Geometry check sheet. Reference: the model listing, model coordinates, mm. Face numbers are marked on the shaded views. A direction names the side the tool comes from. Give positions to 0.01 mm unless a question says otherwise; leave off trailing zeros. Loops run counter-clockwise (first coordinate to the right, second up) from the corner with the lowest first, then second, coordinate; pieces in that order, holes last.
1. Cross-section at D-D, the plane z = 1.25. Record the cut outline in (x, y).
2. Tool access check on the marked faces 1, 2 and 3. Record the directions out of +Z, -Z, +X, -X, +Y, -Y that give a thin tool (end or side, any length) a straight path to the whole face; none if there is none.
3. Cross-section at B-B, the plane y = 20. Record the cut outline in (x, z) (3 decimals).
4. Material ranges on L1, parallel to X at y = 10, z = 9 (3 decimals); L2, parallel to X at y = 14, z = 4; L3, parallel to X at y = 3.75, z = 9.5, recorded low to high.
5. Release check for a two-part mould opening along Z. For the marked faces 4, 5 and 6 record: +Z half, -Z half, draft (parallel to the pull), parting line (faces both ways), or undercut.
6. Cross-section at C-C, the plane x = 48.5. Record the cut outline in (y, z) (3 decimals), plus the area to 3 significant figures.
7. Cross-section at A-A, the plane z = 9. State how many separate pieces and enclosed holes the cut face has, plus the area to 3 significant figures.
from build123d import *

# Parameters (mm, degrees)
SKETCH1_W           = 75
SKETCH1_H           = 18
BOSS_EXTRUDE1_DEPTH = 24
SKETCH2_W           = 36
SKETCH2_H           = 18
CUT_EXTRUDE1_DEPTH  = 20
CUT_EXTRUDE2_REACH  = 81.681
SKETCH3_R           = 2.075
CUT_EXTRUDE4_REACH  = 82.777
SKETCH4_R           = 3.075
CUT_EXTRUDE5_DEPTH  = 5


with BuildPart() as part:
    # Sketch1 → Boss-Extrude1 (new body)
    with BuildSketch(Plane(origin=(0, 0, 0), x_dir=(1, 0, 0), z_dir=(0, 1, 0))):
        with Locations((37.5, -9)):
            Rectangle(SKETCH1_W, SKETCH1_H)
    extrude(amount=BOSS_EXTRUDE1_DEPTH)

    # Sketch2 → Cut-Extrude1 (cut)
    with BuildSketch(Plane(origin=(0, 24, 0), x_dir=(1, 0, 0), z_dir=(0, 1, 0))):
        with Locations((37.5, -9)):
            Rectangle(SKETCH2_W, SKETCH2_H)
    extrude(amount=-CUT_EXTRUDE1_DEPTH, mode=Mode.SUBTRACT)

    # Sketch3 → Cut-Extrude2 (cut, up to next)
    with BuildSketch(Plane(origin=(0, 4, 0), x_dir=(1, 0, 0), z_dir=(0, 1, 0)), mode=Mode.PRIVATE) as cut_extrude2_sk1:
        with Locations(Location((26.5, -9, 0), (0, 0, 270))):
            Circle(SKETCH3_R)
    cut_extrude2_tool1 = extrude(cut_extrude2_sk1.sketch, amount=-CUT_EXTRUDE2_REACH, mode=Mode.PRIVATE) & part.part
    # Sketch3 → Cut-Extrude2 (cut, up to next)
    with BuildSketch(Plane(origin=(0, 4, 0), x_dir=(1, 0, 0), z_dir=(0, 1, 0)), mode=Mode.PRIVATE) as cut_extrude2_sk2:
        with Locations(Location((48.5, -9, 0), (0, 0, 270))):
            Circle(SKETCH3_R)
    cut_extrude2_tool2 = extrude(cut_extrude2_sk2.sketch, amount=-CUT_EXTRUDE2_REACH, mode=Mode.PRIVATE) & part.part
    add(cut_extrude2_tool1.solids().sort_by_distance((26.5, 4, 9))[0], mode=Mode.SUBTRACT)
    add(cut_extrude2_tool2.solids().sort_by_distance((48.5, 4, 9))[0], mode=Mode.SUBTRACT)

    # Sketch4 → Cut-Extrude4 (cut, up to next)
    with BuildSketch(Plane(origin=(0, 24, 0), x_dir=(1, 0, 0), z_dir=(0, 1, 0)), mode=Mode.PRIVATE) as cut_extrude4_sk1:
        with Locations(Location((9.5, -9, 0), (0, 0, 270))):
            Circle(SKETCH4_R)
    cut_extrude4_tool1 = extrude(cut_extrude4_sk1.sketch, amount=-CUT_EXTRUDE4_REACH, mode=Mode.PRIVATE) & part.part
    # Sketch4 → Cut-Extrude4 (cut, up to next)
    with BuildSketch(Plane(origin=(0, 24, 0), x_dir=(1, 0, 0), z_dir=(0, 1, 0)), mode=Mode.PRIVATE) as cut_extrude4_sk2:
        with Locations(Location((65.5, -9, 0), (0, 0, 270))):
            Circle(SKETCH4_R)
    cut_extrude4_tool2 = extrude(cut_extrude4_sk2.sketch, amount=-CUT_EXTRUDE4_REACH, mode=Mode.PRIVATE) & part.part
    add(cut_extrude4_tool1.solids().sort_by_distance((9.5, 24, 9))[0], mode=Mode.SUBTRACT)
    add(cut_extrude4_tool2.solids().sort_by_distance((65.5, 24, 9))[0], mode=Mode.SUBTRACT)

    # Sketch5 → Cut-Extrude5 (cut)
    with BuildSketch(Plane.XZ):
        Polygon((14.5, 11.886751346), (9.5, 14.773502692), (4.5, 11.886751346), (4.5, 6.113248654), (9.5, 3.226497308), (14.5, 6.113248654), align=None)
        Polygon((70.5, 6.113248654), (70.5, 11.886751346), (65.5, 14.773502692), (60.5, 11.886751346), (60.5, 6.113248654), (65.5, 3.226497308), align=None)
    extrude(amount=-CUT_EXTRUDE5_DEPTH, mode=Mode.SUBTRACT)


solid = part.part
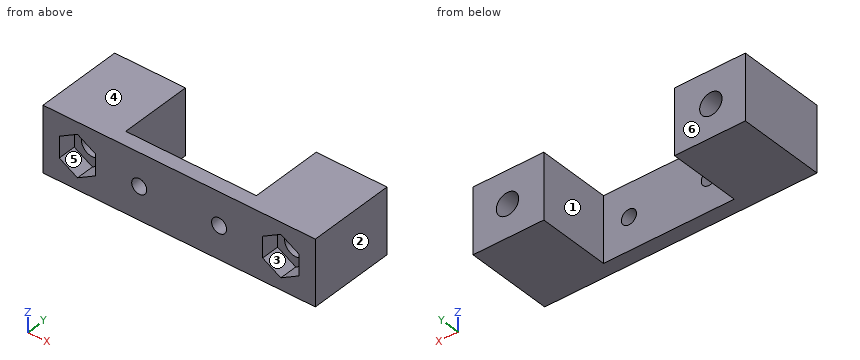
Result:
1. outline: (0, 0) - (75, 0) - (75, 24) - (55.5, 24) - (55.5, 4) - (19.5, 4) - (19.5, 24) - (0, 24) - close
2. face 1: +Z, -Z, +Y
2. face 2: +Z, -Z, +X, +Y, -Y
2. face 3: -Y
3. outline: (0, 0) - (19.5, 0) - (19.5, 18) - (0, 18) - close; (55.5, 0) - (75, 0) - (75, 18) - (55.5, 18) - close; hole circle Ø6.15 at (9.5, 9); hole circle Ø6.15 at (65.5, 9)
4. L1: x = 0 to 6.425, 12.575 to 19.5, 55.5 to 62.425, 68.575 to 75
4. L2: x = 0 to 19.5, 55.5 to 75
4. L3: x = 0 to 4.5, 14.5 to 24.49, 28.51 to 46.49, 50.51 to 60.5, 70.5 to 75
5. face 4: +Z half
5. face 5: undercut
5. face 6: draft
6. outline: (0, 0) - (4, 0) - (4, 6.925) - (0, 6.925) - close; (0, 11.075) - (4, 11.075) - (4, 18) - (0, 18) - close
6. area: 55.4 mm2
7. separate pieces: 5
7. enclosed holes: 0
7. area: 713 mm2
